from build123d import *

# Parameters (mm, degrees)
F0_R     = 63.5
F0_R_2   = 50.8
F0_W     = 13.716
F0_H     = 7.8232
F1_DEPTH = 76.2
F2_DEPTH = 25.4
F3_DEPTH = 127


with BuildPart() as f1:
    # F0 (on Front) → F1 (new body)
    with BuildSketch(Plane.XZ):
        Circle(F0_R)
        Circle(F0_R_2, mode=Mode.SUBTRACT)
        with Locations((0, 56.898177)):
            Rectangle(F0_W, F0_H, mode=Mode.SUBTRACT)
    extrude(amount=F1_DEPTH)

    # F0 (on Front) → F2 (join)
    with BuildSketch(Plane.XZ):
        Circle(F0_R_2)
    extrude(amount=F2_DEPTH)

    # F0 (on Front) → F3 (join)
    with BuildSketch(Plane.XZ):
        with Locations((0, 56.898177)):
            Rectangle(F0_W, F0_H)
    extrude(amount=F3_DEPTH)


solid = f1.part
Design review of the part built by this model. Coordinates are the model's own, in mm. A direction names the side the tool comes from. Round coordinates to 2 decimals unless told otherwise and drop trailing zeros. Loops run counter-clockwise (first coordinate to the right, second up) from the corner with the lowest first, then second, coordinate; pieces in that order, holes last. Notation, with made-up numbers: (15, 51) -> (58, 51) arc R26 cw to (58, 86) -> close; hole circle Ø8 at (84, -34.5). An arc over 180 degrees is marked (long way). Use one line per item in the form item = value. Start each with the question number.
Q1. We need section A-A on z = 0. Give the boundary of the cut face in (x, y), then the cut area to 3 significant figures.
Q2. Machinability: for faces 1 (the face through (0, -101, 52.987)), 2 (the face through (-1, -25.4, 1)), 3 (the face through (-6.858, -101, 57)), which of the approach directions +Z, -Z, +X, -X, +Y, -Y give a long, thin tool a straight path to every point of the face, cutting with its end or side? Answer none if there is none.
Q3. For pin 1 Ø7 at (x, y) = (2, -97) entering from +Z; pin 2 Ø2 at (x, z) = (-47.5, -11.5) entering from -Y; pin 3 Ø12 at (y, z) = (-58.5, 33) entering from +X, all flat-tipped, find the tip position at first contact; note any pin that passes through.
Q4. We need section B-B on y = -47. Give the boundary of the cut face in (x, z).
Q5. We need section C-C on x = 0. Give the boundary of the cut face in (y, z).
Q6. We need section D-D on y = -22. Give the boundary of the cut face in (x, z).
Q7. Draft analysis for pull direction X (two halves, no side actions). For faces 4 (the face through (-11.012, -50.444, -49.592)), 5 (the face through (-43, -76.2, 29)), 6 (the face through (6.858, -101, 57)), state which applies: +X half, -X half, draft (parallel to the pull), parting line (faces both ways), or undercut.
Q8. Wall thickness on line 1 along Z through (x, y) = (0, -51); line 2 along X through (y, z) = (-66.5, 39); line 3 along Z through (x, y) = (-32.5, -66): over which ranges is each line inside the solid? List them lowest first. Write a range as [from, to].
Calculated:
q1.outline = (-63.5, -76.2) -> (-50.8, -76.2) -> (-50.8, -25.4) -> (50.8, -25.4) -> (50.8, -76.2) -> (63.5, -76.2) -> (63.5, 0) -> (-63.5, 0) -> close
q1.area = 4,520 mm²
q2.face_1 = -Z, +X, -X, -Y
q2.face_2 = -Y
q2.face_3 = +Z, -Z, -X, -Y
q3.pin_1 = 60.81
q3.pin_2 = -25.4
q3.pin_3 = 57.47
q4.outline = circle Ø127 at (0, 0); hole circle Ø101.6 at (0, 0)
q5.outline = (-127, 52.99) -> (-76.2, 52.99) -> (-76.2, 50.8) -> (-25.4, 50.8) -> (-25.4, -50.8) -> (-76.2, -50.8) -> (-76.2, -63.5) -> (0, -63.5) -> (0, 63.5) -> (-76.2, 63.5) -> (-76.2, 60.81) -> (-127, 60.81) -> close
q6.outline = circle Ø127 at (0, 0)
q7.face_4 = undercut
q7.face_5 = draft
q7.face_6 = +X half
q8.line_1 = [-63.5, -50.8], [50.8, 63.5]
q8.line_2 = [-50.11, -32.55], [32.55, 50.11]
q8.line_3 = [-54.55, -39.04], [39.04, 54.55]
